Read the model definition and answer for the solid it produces. Units are mm, in the model's axes. Face numbers are marked on the shaded views. Coordinates: 2 decimals unless noted, no trailing zeros. Write each loop counter-clockwise with the first axis right and the second up, starting at its lowest first coordinate (ties: lowest second). Pieces come first, ordered by that corner, then holes. Notation, with made-up numbers: (72.5, 79) -> (90.5, 79) arc R19 ccw to (90.5, 100) -> close; hole circle Ø7 at (-19, 15). An arc over 180 degrees is marked (long way). Use CSV: the item, a comma, the result in double quotes.
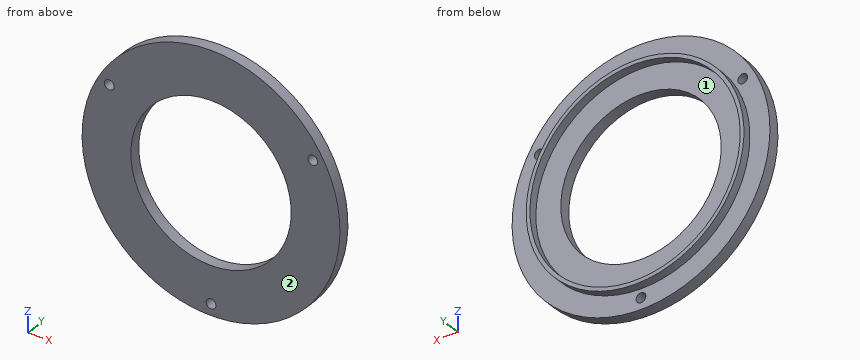
from build123d import *

# Parameters (mm, degrees)
SKETCH1_R                          = 45
SKETCH1_R_2                        = 28
COLLAR_ANNULUS_OD90_ID56_T4_DEPTH  = 4
SKETCH2_R                          = 38
SKETCH2_R_2                        = 36.7
RETAINING_RIM_OD76_ID73_4_H3_DEPTH = 3
MOUNTING_HOLES_3X_3_4_PCD82_D      = 3.4


with BuildPart() as part:
    # Sketch1 → Collar_Annulus_OD90_ID56_T4 (new body)
    with BuildSketch(Plane(origin=(0, 0, 0), x_dir=(1, 0, 0), z_dir=(0, 1, 0))):
        with Locations(Location((0, 0, 0), (0, 0, 270))):
            Circle(SKETCH1_R)
        with Locations(Location((0, 0, 0), (0, 0, 270))):
            Circle(SKETCH1_R_2, mode=Mode.SUBTRACT)
    extrude(amount=COLLAR_ANNULUS_OD90_ID56_T4_DEPTH)

    # Sketch2 → Retaining_Rim_OD76_ID73.4_H3 (add)
    with BuildSketch(Plane(origin=(0, 4, 0), x_dir=(1, 0, 0), z_dir=(0, 1, 0))):
        with Locations(Location((0, 0, 0), (0, 0, 270))):
            Circle(SKETCH2_R)
        with Locations(Location((0, 0, 0), (0, 0, 270))):
            Circle(SKETCH2_R_2, mode=Mode.SUBTRACT)
    extrude(amount=RETAINING_RIM_OD76_ID73_4_H3_DEPTH)

    # Mounting_Holes_3xØ3.4_PCD82 (through all)
    with Locations(Plane(origin=(0, 4, 0), x_dir=(1, 0, 0), z_dir=(0, 1, 0))):
        with Locations((-35.507041555, -20.5), (0, 41), (35.507041555, -20.5)):
            Hole(MOUNTING_HOLES_3X_3_4_PCD82_D / 2)


solid = part.part
1. A cutting plane is placed at A-A (z = 0). Give the vertices of the cut face in (x, y), and give its area (3 significant figures).
Solutions:
outline,"(-45, 0) -> (-28, 0) -> (-28, 4) -> (-36.7, 4) -> (-36.7, 7) -> (-38, 7) -> (-38, 4) -> (-45, 4) -> close; (28, 0) -> (45, 0) -> (45, 4) -> (38, 4) -> (38, 7) -> (36.7, 7) -> (36.7, 4) -> (28, 4) -> close"
area,"144 mm^2"
2. For a pull along Z with two mould halves and no side action, classify the marked faces 1 and 2 as pulls with the +Z half, pulls with the -Z half, needs draft (parallel to the pull), parting line crosses it, or undercut.
Solutions:
face 1,"undercut"
face 2,"needs draft"
3. Each of these flat-tipped pins is pushed along its axis until it touches: pin 1 Ø3 at (x, z) = (35.51, 20.5) entering from -Y; pin 2 Ø2 at (x, z) = (-16.5, 27) entering from +Y; pin 3 Ø2 at (y, z) = (6, 19.5) entering from +X; pin 4 Ø2 at (y, z) = (1, 10.5) entering from +X. Where does it stop, or does it pass through?
Solutions:
pin 1,"passes through"
pin 2,"stops at y = 4"
pin 3,"stops at x = 33.19"
pin 4,"stops at x = 43.99"
4. A cutting plane is placed at D-D (z = 20.5). Give the vertices of the cut face in (x, y).
Solutions:
outline,"(-40.06, 0) -> (-37.21, 0) -> (-37.21, 4) -> (-40.06, 4) -> close; (-33.81, 0) -> (-19.07, 0) -> (-19.07, 4) -> (-30.44, 4) -> (-30.44, 7) -> (-32, 7) -> (-32, 4) -> (-33.81, 4) -> close; (19.07, 0) -> (33.81, 0) -> (33.81, 4) -> (32, 4) -> (32, 7) -> (30.44, 7) -> (30.44, 4) -> (19.07, 4) -> close; (37.21, 0) -> (40.06, 0) -> (40.06, 4) -> (37.21, 4) -> close"
5. Find the intervals of material crossed by line 1 along X through (y, z) = (2.15, 20.5); line 2 along X through (y, z) = (1.05, 0); line 3 along Y through (x, z) = (-33.5, 20.5), in increasing order.
Solutions:
line 1,"x = -40.06 to -37.21, -33.81 to -19.07, 19.07 to 33.81, 37.21 to 40.06"
line 2,"x = -45 to -28, 28 to 45"
line 3,"y = 0 to 4"
6. A cutting plane is placed at B-B (y = 1.5). Give the vertices of the cut face in (x, z).
Solutions:
outline,"circle Ø90 at (0, 0); hole circle Ø3.4 at (-35.51, 20.5); hole circle Ø56 at (0, 0); hole circle Ø3.4 at (0, -41); hole circle Ø3.4 at (35.51, 20.5)"
7. A cutting plane is placed at C-C (x = -7). Give the vertices of the cut face in (y, z).
Solutions:
outline,"(0, -44.45) -> (4, -44.45) -> (4, -37.35) -> (7, -37.35) -> (7, -36.03) -> (4, -36.03) -> (4, -27.11) -> (0, -27.11) -> close; (0, 27.11) -> (4, 27.11) -> (4, 36.03) -> (7, 36.03) -> (7, 37.35) -> (4, 37.35) -> (4, 44.45) -> (0, 44.45) -> close"
